Part model, mm, in its own coordinate system. A direction names the side the tool comes from. Coordinates: 2 decimals unless noted, no trailing zeros. Loops run counter-clockwise (first coordinate to the right, second up) from the corner with the lowest first, then second, coordinate; pieces in that order, holes last. Notation, with made-up numbers: M 55.5,2 L 80.5,2 A23 ccw 80.5,30 Z; hole C 36.5,59 d11. An arc over 180 degrees is marked long. Use CSV: the item, a comma, the result in double quotes. Start each with the question number.
from build123d import *

# Parameters (mm, degrees)
SKETCH1_W           = 16.9
SKETCH1_H           = 11.7
BOSS_EXTRUDE1_DEPTH = 5
SKETCH2_W           = 11.05
SKETCH2_H           = 5.85
CUT_EXTRUDE1_DEPTH  = 0.95
SKETCH3_W           = 10.2
SKETCH3_H           = 5.1
CUT_EXTRUDE2_DEPTH  = 3
SKETCH4_W           = 10.2
SKETCH4_H           = 5.1
BOSS_EXTRUDE2_DEPTH = 1
BOSS_EXTRUDE3_DEPTH = 176
SKETCH6_W           = 26.9
SKETCH6_H           = 26.95
BOSS_EXTRUDE4_DEPTH = 2
CHAMFER1_SIZE       = 14
CHAMFER1_SIZE2      = 7.443932043


with BuildPart() as part:
    # Sketch1 → Boss-Extrude1 (new body)
    with BuildSketch(Plane(origin=(0, 0, 0), x_dir=(1, 0, 0), z_dir=(0, 1, 0))):
        with Locations((8.45, 5.85)):
            Rectangle(SKETCH1_W, SKETCH1_H)
    extrude(amount=BOSS_EXTRUDE1_DEPTH)

    # Sketch2 → Cut-Extrude1 (cut)
    with BuildSketch(Plane.XZ):
        with Locations((8.45, -5.85)):
            Rectangle(SKETCH2_W, SKETCH2_H)
    extrude(amount=-CUT_EXTRUDE1_DEPTH, mode=Mode.SUBTRACT)

    # Sketch3 → Cut-Extrude2 (cut)
    with BuildSketch(Plane.XZ.offset(-0.95)):
        with Locations((8.475, -5.875)):
            Rectangle(SKETCH3_W, SKETCH3_H)
    extrude(amount=-CUT_EXTRUDE2_DEPTH, mode=Mode.SUBTRACT)

    # Sketch4 → Boss-Extrude2 (add)
    with BuildSketch(Plane.XZ.offset(-0.95)):
        with Locations((8.475, -5.875)):
            Rectangle(SKETCH4_W, SKETCH4_H)
    extrude(amount=-BOSS_EXTRUDE2_DEPTH)

    # Sketch5 → Boss-Extrude3 (add)
    with BuildSketch(Plane(origin=(0, 5, 0), x_dir=(1, 0, 0), z_dir=(0, 1, 0))):
        Polygon((2, 0), (2, 2), (7.2, 2), (7.2, 9.7), (9.7, 9.7), (9.7, 2), (14.9, 2), (14.9, 0), align=None)
    extrude(amount=BOSS_EXTRUDE3_DEPTH)

    # Sketch6 → Boss-Extrude4 (add)
    with BuildSketch(Plane.XY):
        with Locations((8.45, 167.525)):
            Rectangle(SKETCH6_W, SKETCH6_H)
    extrude(amount=-BOSS_EXTRUDE4_DEPTH)

    # Chamfer1
    chamfer1_edges = [part.edges().sort_by_distance(p)[0] for p in [
        (8.45, 181, -9.7),
    ]]
    chamfer1_side = [part.faces().sort_by_distance(p)[0] for p in [
        (8.45, 93, -9.7),
    ]]
    chamfer(chamfer1_edges, length=CHAMFER1_SIZE, length2=CHAMFER1_SIZE2, reference=chamfer1_side[0])


solid = part.part
1. Tool access for faces 4 (the face through (0, 2, -6)), 5 (the face through (4, 94, -2)), 6 (the face through (9.7, 92, -6)): list every direction of +Z, -Z, +X, -X, +Y, -Y with a clear straight run to the whole face (end or side of a thin tool).
2. Slice it at A-A, the plane y = 165.5. List the corners of the cut face in (x, z).
3. Slice it at B-B, the plane x = -2.5. List the corners of the cut face in (y, z), and give its area (3 significant figures).
4. Pin check, flat tips, straight feed: pin 1 (12 mm diameter, centred on x = 8, y = 47.5, fed in from -Z); pin 2 (1.5 mm diameter, centred on y = 37.5, z = -7.5, fed in from -X); pin 3 (0.8 mm diameter, centred on y = 0.5, z = -7, fed in from -X). Stop position of each tip, or through.
5. Two-plate mould, pull along Z, no slides. Class faces 1 (the face through (7.2, 92, -6)), 2 (the face through (8, 92, 0)), 3 (the face through (8, 0.95, -6)): pulls with the +Z half, pulls with the -Z half, needs draft (parallel to the pull), parting line crosses it, or undercut.
6. Slice it at D-D, the plane y = 55.5. List the corners of the cut face in (x, z), and give its area (4 significant figures).
7. Slice it at C-C, the plane z = -5.5. List the corners of the cut face in (x, y) (3 decimals).
8. Wall check: probe 1 along Y at (x, z) = (10, -8); probe 2 along X at (y, z) = (46, -2.25); probe 3 along Y at (x, z) = (12, -11). Give the ranges that are in metal, low to high.
Found:
1,face 4,"+Z, -Z, -X, -Y"
1,face 5,"-Z, -X, +Y"
1,face 6,"-Z, +X, +Y"
2,outline,"M -5,-2 L 7.2,-2 L 7.2,-9.7 L 9.7,-9.7 L 9.7,-2 L 21.9,-2 L 21.9,0 L -5,0 Z"
3,outline,"M 154.05,-2 L 181,-2 L 181,0 L 154.05,0 Z"
3,area,"53.9 mm^2"
4,pin 1,"z = -9.7"
4,pin 2,"x = 7.2"
4,pin 3,"x = 0"
5,face 1,"needs draft"
5,face 2,"pulls with the +Z half"
5,face 3,"undercut"
6,outline,"M 2,-2 L 7.2,-2 L 7.2,-9.7 L 9.7,-9.7 L 9.7,-2 L 14.9,-2 L 14.9,0 L 2,0 Z"
6,area,"45.05 mm^2"
7,outline,"M 0,0 L 2.925,0 L 2.925,0.95 L 13.975,0.95 L 13.975,0 L 16.9,0 L 16.9,5 L 9.7,5 L 9.7,174.899 L 7.2,174.899 L 7.2,5 L 0,5 Z; hole M 3.375,1.95 L 13.575,1.95 L 13.575,3.95 L 3.375,3.95 Z"
8,probe 1,"0.95 to 1.95, 3.95 to 5"
8,probe 2,"7.2 to 9.7"
8,probe 3,"0 to 5"
